Can you work these out from the drawing? Everything is in mm from the part's minimum corner. A direction names the side the tool comes from. Round coordinates to 2 decimals unless told otherwise and drop trailing zeros. Order: outer loops, then holes, each group sorted by start corner. A loop starts at its lowest first (then second) coordinate and runs counter-clockwise, first axis right, second up. Notation, with made-up numbers: (21.25, 87.5) -> (32.25, 87.5) arc R8 cw to (32.25, 92.5) -> close; hole circle Ø3 at (38, 34.5). An arc over 180 degrees is marked (long way). One line per item, written item: value.
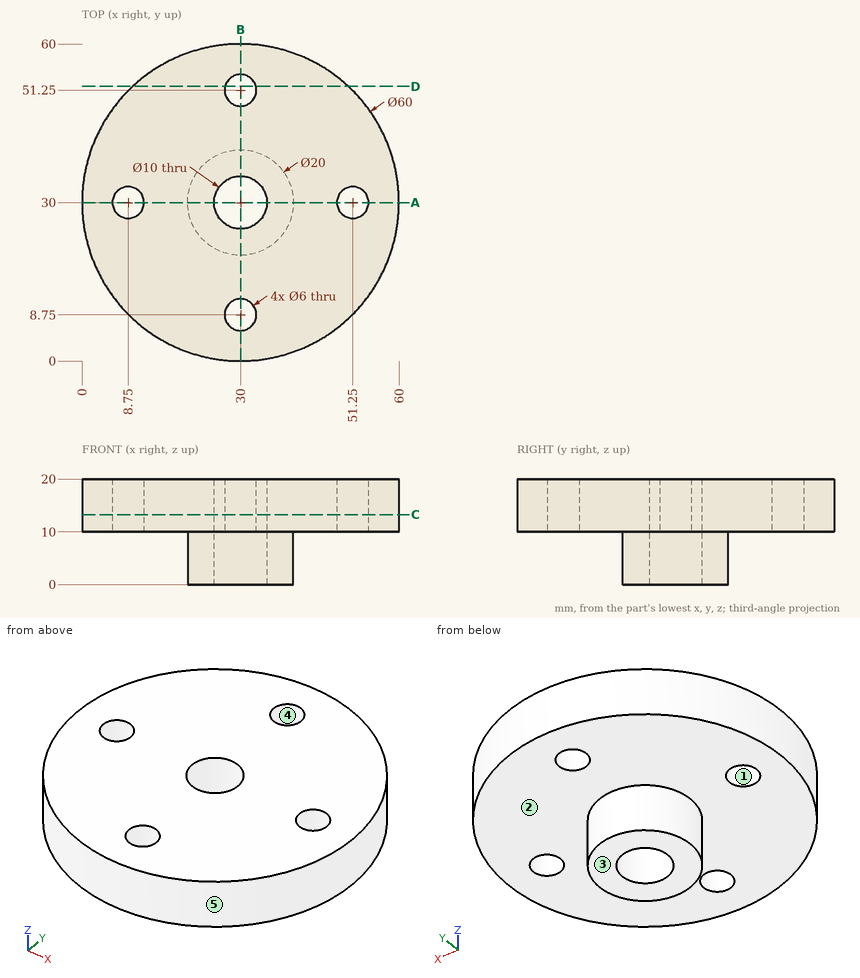
Q1. We'd pull the mould along X, two halves only. Please class the marked faces 3, 4 and 5: released by +X, released by -X, zero draft, split by the parting line, or undercut.
Answers below:
face 3: zero draft
face 4: undercut
face 5: split by the parting line
Q2. I want a section at C-C on z = 13.25. List the corners of the cut face in (x, y) for me, plus the area to 3 significant figures.
Answers below:
outline: circle Ø60 at (30, 30); hole circle Ø6 at (8.75, 30); hole circle Ø10 at (30, 30); hole circle Ø6 at (30, 8.75); hole circle Ø6 at (30, 51.25); hole circle Ø6 at (51.25, 30)
area: 2,640 mm^2
Q3. I want a section at D-D on y = 52. List the corners of the cut face in (x, z) for me.
Answers below:
outline: (9.6, 10) -> (27.1, 10) -> (27.1, 20) -> (9.6, 20) -> close; (32.9, 10) -> (50.4, 10) -> (50.4, 20) -> (32.9, 20) -> close
Q4. Will these pins go through, and if not, where does the flat tip stop? pin 1 Ø6 at (x, y) = (9, 23) entering from -Z; pin 2 Ø5 at (y, z) = (23.5, 13) entering from +X; pin 3 Ø1.5 at (y, z) = (43, 14) entering from -X (3 decimals).
Answers below:
pin 1: z = 10
pin 2: x = 59.73
pin 3: x = 2.615
Q5. I want a section at A-A on y = 30. List the corners of the cut face in (x, z) for me, plus the area to 3 significant figures.
Answers below:
outline: (0, 10) -> (5.75, 10) -> (5.75, 20) -> (0, 20) -> close; (11.75, 10) -> (20, 10) -> (20, 0) -> (25, 0) -> (25, 20) -> (11.75, 20) -> close; (35, 0) -> (40, 0) -> (40, 10) -> (48.25, 10) -> (48.25, 20) -> (35, 20) -> close; (54.25, 10) -> (60, 10) -> (60, 20) -> (54.25, 20) -> close
area: 480 mm^2
Q6. On a 3-axis mill with a long thin cutter (end or side, diameter ignored), from which of +Z, -Z, +X, -X, +Y, -Y can I reach the whole of each face in a straight line? I mean the marked faces 1 and 2. Say none if no direction works.
Answers below:
face 1: +Z, -Z
face 2: -Z
Q7. Please list where these lines run through material, in increasing order: line 1 along Z through (x, y) = (43, 14); line 2 along Y through (x, z) = (25.5, 6.5); line 3 along Y through (x, z) = (8.75, 16).
Answers below:
line 1: 10 to 20
line 2: 21.07 to 27.82, 32.18 to 38.93
line 3: 8.82 to 27, 33 to 51.18
